```python
from build123d import *

# Parameters (mm, degrees)
SKETCH1_R                          = 7.9375
SKETCH1_R_2                        = 6.437500000000001
PIPE_CONFIGURED_21_3_X_2_3_3_DEPTH = 522.055690959
ESBO_O11_R                         = 7.937500000000085
ESBO_O12_R                         = 7.937500000000085


with BuildPart() as part:
    # Sketch1 → Pipe - configured 21.3 X 2.3(3) (new body)
    with BuildSketch(Plane(origin=(854.3898367144717, 250, -261.0278454796051), x_dir=(1, 0, 0), z_dir=(0, 0, 1))):
        Circle(SKETCH1_R)
        Circle(SKETCH1_R_2, mode=Mode.SUBTRACT)
    extrude(amount=PIPE_CONFIGURED_21_3_X_2_3_3_DEPTH)

    # Varredura de corte1: sweep along a curve in space
    with BuildLine() as varredura_de_corte1_path:
        Line((910.0000000000001, 0, 265), (910.0000000000001, 139.26905749604418, 265))
        ThreePointArc((910.0000000000001, 139.26905749604418, 265), (908.6404967596997, 149.62181930014503, 264.9028926256928), (904.6546349379392, 159.26905749604424, 264.61818820985286))
        Line((904.6546349379392, 159.26905749604424, 264.61818820985286), (858.6941735437408, 239.0777295619333, 261.3352981102673))
        ThreePointArc((858.6941735437408, 239.0777295619333, 261.3352981102673), (854.2945586384378, 250.42014500440925, 261.02103990274554), (853.500633741435, 262.56395927183974, 260.964330981531))
        Line((853.500633741435, 262.56395927183974, 260.964330981531), (910.0000000000001, 910, 265))
    # Esboço11 → Varredura de corte1 (sweep, cut)
    with BuildSketch(Plane(origin=(0, 0, 0), x_dir=(1, 0, 0), z_dir=(0, 1, 0))):
        with Locations((910.0000000000001, -265)):
            Circle(ESBO_O11_R)
    sweep(path=varredura_de_corte1_path.line, mode=Mode.SUBTRACT)

    # Varredura de corte2: sweep along a curve in space
    with BuildLine() as varredura_de_corte2_path:
        Line((910.0000000000001, 0, -265), (910.0000000000001, 139.26905749604356, -265))
        ThreePointArc((910.0000000000001, 139.26905749604356, -265), (908.6404967596995, 149.62181930014447, -264.9028926256928), (904.6546349379391, 159.26905749604364, -264.6181882098528))
        Line((904.6546349379391, 159.26905749604364, -264.6181882098528), (858.6941735437406, 239.07772956193315, -261.33529811026716))
        ThreePointArc((858.6941735437406, 239.07772956193315, -261.33529811026716), (854.2945586384376, 250.4201450044091, -261.0210399027455), (853.5006337414345, 262.5639592718396, -260.96433098153096))
        Line((853.5006337414345, 262.5639592718396, -260.96433098153096), (910.0000000000001, 910, -265))
    # Esboço12 → Varredura de corte2 (sweep, cut)
    with BuildSketch(Plane(origin=(0, 0, 0), x_dir=(1, 0, 0), z_dir=(0, 1, 0))):
        with Locations((910.0000000000001, 265)):
            Circle(ESBO_O12_R)
    sweep(path=varredura_de_corte2_path.line, mode=Mode.SUBTRACT)


solid = part.part
```
Geometry check sheet. Reference: the model listing, model coordinates, mm. Give positions to 0.01 mm unless a question says otherwise; leave off trailing zeros. Write each loop counter-clockwise with the first axis right and the second up, starting at its lowest first coordinate (ties: lowest second). Pieces come first, ordered by that corner, then holes. Notation, with made-up numbers: (49, 62) -> (108, 62) arc R26 ccw to (108, 84) -> close; hole circle Ø5 at (65, 80.5). An arc over 180 degrees is marked (long way). One line per question, with ' | ' between items.
Item 1: Depth check by flat-ended pin: pin 1 (4 mm diameter, centred on y = 256.5, z = -88.5, fed in from +X); pin 2 (2 mm diameter, centred on x = 859.5, z = 203, fed in from +Y); pin 3 (1 mm diameter, centred on x = 850.5, y = 254, fed in from +Z); pin 4 (8 mm diameter, centred on x = 851, z = -19.5, fed in from -Y). Enter the tip coordinate at first touch or a pass-through.
Determined:
pin 1: x = 860.93 | pin 2: y = 256.79 | pin 3: through | pin 4: y = 242.06
Item 2: Sectioned sample at A-A, the plane z = -63.5. Record the boundary of the cut face in (x, y) (1 decimal).
Determined:
outline: circle Ø15.9 at (854.4, 250); hole circle Ø12.9 at (854.4, 250)
Item 3: Scan lines: line 1 along X through (y, z) = (249, 208.5); line 2 along Y through (x, z) = (853.5, -65); line 3 along X through (y, z) = (250, -60.5). Record each from-to range of solid material in increasing order.
Determined:
line 1: 846.52 to 848.03, 860.75 to 862.26 | line 2: 242.11 to 243.62, 256.38 to 257.89 | line 3: 846.45 to 847.95, 860.83 to 862.33
